Build history of the part. All positions in model axes, mm. A direction names the side the tool comes from. Give positions to 0.01 mm unless a question says otherwise; leave off trailing zeros. Order: outer loops, then holes, each group sorted by start corner. A loop starts at its lowest first (then second) coordinate and runs counter-clockwise, first axis right, second up. Notation, with made-up numbers: (19, -37) - (73, -37) arc R32 ccw to (73, -2) - close; hole circle Ø1 at (86, 72). An arc over 180 degrees is marked (long way). One line per item, written item: value.
Autodesk Inventor part; units mm, degrees
ref_plane "YZ Plane" through (0, 0, 0) normal (1, 0, 0) x (0, 1, 0)
ref_plane "XZ Plane" through (0, 0, 0) normal (0, 1, 0) x (-1, 0, 0)
ref_plane "XY Plane" through (0, 0, 0) normal (0, 0, 1) x (1, 0, 0)
sketch "Sketch1" plane through (0, 0, 0) normal (0, 0, 1) x (1, 0, 0)
  line L0 (-30.1625, -17.4625) -> (30.1625, -17.4625) construction
  line L1 (30.1625, -17.4625) -> (30.1625, 17.4625) construction
  line L2 (30.1625, 17.4625) -> (-30.1625, 17.4625) construction
  line L3 (-30.1625, 17.4625) -> (-30.1625, -17.4625) construction
  line L4 (-30.1625, -17.4625) -> (30.1625, 17.4625) construction
  line L5 (30.1625, -17.4625) -> (-30.1625, 17.4625) construction
  circle A0 centre (-30.1625, -17.4625) radius 6.35 construction
  circle A1 centre (-30.1625, 17.4625) radius 6.35 construction
  circle A2 centre (30.1625, 17.4625) radius 6.35 construction
  circle A3 centre (30.1625, -17.4625) radius 6.35 construction
  circle A4 centre (0, 0) radius 22.225 construction
  arc A5 (29.4959, -23.7774) -> (-29.4959, -23.7774) centre (0, -303.2125) ccw
  arc A6 (32.7003, 11.6417) -> (32.7003, -11.6417) centre (37.7759, 0) ccw
  arc A7 (-29.4959, 23.7774) -> (29.4959, 23.7774) centre (0, 303.2125) ccw
  arc A8 (-32.7003, -11.6417) -> (-32.7003, 11.6417) centre (-37.7759, 0) ccw
  arc A9 (-31.4314, -14.5521) -> (-31.4314, 14.5521) centre (-37.7759, 0) ccw
  arc A10 (184.3591, -86.9718) -> (-184.3591, -86.9718) centre (0, -303.2125) ccw
  arc A11 (31.4314, 14.5521) -> (31.4314, -14.5521) centre (37.7759, 0) ccw
  arc A12 (-184.3591, 86.9718) -> (184.3591, 86.9718) centre (0, 303.2125) ccw
  arc A13 (-29.4959, 23.7774) -> (-32.7003, 11.6417) centre (-30.1625, 17.4625) ccw
  arc A14 (-27.2047, 11.8434) -> (-24.3854, 20.0982) centre (-30.1625, 17.4625) ccw
  arc A15 (32.7003, 11.6417) -> (29.4959, 23.7774) centre (30.1625, 17.4625) ccw
  arc A16 (24.3854, 20.0982) -> (27.2047, 11.8434) centre (30.1625, 17.4625) ccw
  arc A17 (29.4959, -23.7774) -> (32.7003, -11.6417) centre (30.1625, -17.4625) ccw
  arc A18 (27.2047, -11.8434) -> (24.3854, -20.0982) centre (30.1625, -17.4625) ccw
  arc A19 (-32.7003, -11.6417) -> (-29.4959, -23.7774) centre (-30.1625, -17.4625) ccw
  arc A20 (-24.3854, -20.0982) -> (-27.2047, -11.8434) centre (-30.1625, -17.4625) ccw
  dimension "d0" = 60.325
  dimension "d1" = 34.925
  dimension "d2" = 12.7
  dimension "d3" = 12.7
  dimension "d4" = 12.7
  dimension "d5" = 12.7
  dimension "d6" = 44.45
  dimension "d7" = 12.7
  dimension "d8" = 12.7
  dimension "d9" = 3.175
  dimension "d10" = 3.175
extrude "Extrusion1" add sketch "Sketch1" along normal blind 20.6248 contours A5 A19 A10 A17 | A10 A18 A11 A16 A12 A15 A6 A17 | A19 A8 A13 A12 A14 A9 A20 A10 | A12 A13 A7 A15
fillet "Fillet1" radius 3.175 8 edges at (-27.2047, -11.8434, 10.3124) (-27.2047, 11.8434, 10.3124) (-24.3854, 20.0982, 10.3124) (24.3854, 20.0982, 10.3124) (27.2047, 11.8434, 10.3124) (27.2047, -11.8434, 10.3124) (24.3854, -20.0982, 10.3124) (-24.3854, -20.0982, 10.3124)
hole "Hole1" at (30.1625, 17.4625, 0) at (30.1625, -17.4625, 0) at (-30.1625, -17.4625, 0) at (-30.1625, 17.4625, 0) direction (0, 0, 1) diameter 5.1054 end through all
sketch "Sketch3" plane through (0, 0, 20.6248) normal (0, 0, 1) x (1, 0, 0)
  circle A0 centre (0, 0) radius 24.003
  dimension "d21" = 48.006
extrude "Extrusion2" cut sketch "Sketch3" against normal blind 3.81
equation "\"d8\" = d7"
equation "\"d10\" = d9"
properties part number "AR-011" material "Aluminum 6061"
(1) Drill centre lines: line 1 (Y direction, x = 2, z = 9.5); line 2 (X direction, y = 16, z = 8); line 3 (Y direction, x = 31, z = 13.5). Where is each one in solid material? Low to high.
Completed:
line 1: -22.23 to -19.06, 19.06 to 22.23
line 2: -36.34 to -32.25, -28.07 to -23.98, 23.98 to 28.07, 32.25 to 36.34
line 3: -23.76 to -19.87, -15.05 to -10.74, 10.74 to 15.05, 19.87 to 23.76
(2) Slice it at B-B, the plane x = -6. Give the cut face in (y, z), and give its area (3 significant figures).
Completed:
outline: (-22.29, 0) - (-19.11, 0) - (-19.11, 16.81) - (-22.29, 16.81) - close; (19.11, 0) - (22.29, 0) - (22.29, 16.81) - (19.11, 16.81) - close
area: 107 mm²
(3) Slice it at A-A, the plane y = -2.5. Give the cut face in (x, z).
Completed:
outline: (-25.32, 0) - (-22.1, 0) - (-22.1, 16.81) - (-23.87, 16.81) - (-23.87, 20.62) - (-25.32, 20.62) - close; (22.1, 0) - (25.32, 0) - (25.32, 20.62) - (23.87, 20.62) - (23.87, 16.81) - (22.1, 16.81) - close
(4) Pin check, flat tips, straight feed: P1, Ø4.5, axis at x = 30.16, y = -17.46, coming from the +Z side; P2, Ø3, axis at x = -21.5, y = -1, coming from the -Z side; P3, Ø8, axis at y = 4, z = 15, coming from the -X side; P4, Ø3.5, axis at x = -3, y = -20, coming from the +Z side. Stop position of each tip, or through.
Completed:
P1: through
P2: z = 0
P3: x = -27.91
P4: z = 16.81
(5) 3-axis set-ups, long thin cutter, end or side, ignore diameter. For faces 4 (the face through (25.078, -0.206, 10.168)), 5 (the face through (0, -21, 16.815)), 6 (the face through (24.25, -15.15, 10.17)): which of +Z, -Z, +X, -X, +Y, -Y reach the whole face in a straight line?
Completed:
face 4: +Z, -Z, +X
face 5: +Z
face 6: +Z, -Z
(6) Slice it at C-C, the plane z = 19. Count the separate pieces of the cut face and the enclosed holes in it, and give its area (3 significant figures).
Completed:
separate pieces: 2
enclosed holes: 4
area: 755 mm²
(7) Pull direction Y, two halves, no side cores. Call faces 1 (the face through (0.29, 19.05, 7.88)), 2 (the face through (-0.2, -19.3, 0)), 3 (the face through (0.414, 22.225, 10.168)): +Y half, -Y half, draft (parallel to the pull), parting line (faces both ways), or undercut.
Completed:
face 1: undercut
face 2: draft
face 3: +Y half
